Can you work these out from the model? Positions are in its coordinate system, mm. A direction names the side the tool comes from. Give positions to 0.01 mm unless a question says otherwise; leave off trailing zeros. Write each loop counter-clockwise with the first axis right and the second up, starting at its lowest first coordinate (ties: lowest second). Pieces come first, ordered by that corner, then holes. Notation, with made-up numbers: M 86.25,-31 L 131.25,-31 A19 cw 131.25,-12 Z; hole C 18,37.5 d3. An arc over 180 degrees is marked long. Use CSV: the item, a comma, the result in double quotes. Start each with the question number.
from build123d import *

# Parameters (mm, degrees)
EXTRUDE_2_DEPTH          = 35
EXTRUDE_START            = -100
SKETCH_3_W               = 70
SKETCH_3_H               = 70
EXTRUDE_3_DEPTH          = 10
CUT_EXTRUDE_START        = 35
SKETCH_4_W               = 29.4
SKETCH_4_H               = 90
CUT_EXTRUDE_1_DEPTH      = 25
CHAMFER_1_SIZE           = 10
EXTRUDE_4_DEPTH          = 15
CHAMFER_2_SIZE           = 5
CUT_EXTRUDE_2_DEPTH      = 131.096118313
CUT_EXTRUDE_2_DEPTH_BACK = 131.096118313
SKETCH_6_R               = 2
FILLET_2_R               = 8


with BuildPart() as part:
    # 草图2 → 凸台-拉伸2 (new body)
    with BuildSketch(Plane.XY):
        Polygon((-45, 7.5), (45, 7.5), (45, -12), (40, -12), (40, 0), (14.7, 0), (14.7, -100), (-14.7, -100), (-14.7, 0), (-40, 0), (-40, -12), (-45, -12), align=None)
    extrude(amount=EXTRUDE_2_DEPTH)

    # 草图3 → 凸台-拉伸3 (add)
    with BuildSketch(Plane(origin=(0, 0, 0), x_dir=(1, 0, 0), z_dir=(0, 1, 0)).offset(EXTRUDE_START)):
        with Locations((0, -35)):
            Rectangle(SKETCH_3_W, SKETCH_3_H)
    extrude(amount=EXTRUDE_3_DEPTH)

    # 草图4 → 切除-拉伸1 (cut)
    with BuildSketch(Plane.XY.offset(CUT_EXTRUDE_START)):
        with Locations((0, -45)):
            Rectangle(SKETCH_4_W, SKETCH_4_H)
    extrude(amount=-CUT_EXTRUDE_1_DEPTH, mode=Mode.SUBTRACT)

    # 倒角1
    chamfer_1_edges = [part.edges().sort_by_distance(p)[0] for p in [
        (0, 0, 10),
        (0, -90, 10),
    ]]
    chamfer(chamfer_1_edges, length=CHAMFER_1_SIZE)

    # 草图5 → 凸台-拉伸4 (add)
    with BuildSketch(Plane.XY):
        Polygon((40, -12), (45, -12), (45, 7.5), (-45, 7.5), (-45, -12), (-40, -12), (-40, 0), (40, 0), align=None)
    extrude(amount=-EXTRUDE_4_DEPTH)

    # 倒角2
    chamfer_2_edges = [part.edges().sort_by_distance(p)[0] for p in [
        (0, 0, 0),
    ]]
    chamfer(chamfer_2_edges, length=CHAMFER_2_SIZE)

    # 草图6 → 切除-拉伸2 (cut, two sides: drawn at the far end of the back side and taken through both)
    with BuildSketch(Plane(origin=(0, 0, 0), x_dir=(0, 0, -1), z_dir=(1, 0, 0)).offset(-CUT_EXTRUDE_2_DEPTH_BACK)):
        with Locations((10, -6)):
            Circle(SKETCH_6_R)
        with Locations((-25, -6)):
            Circle(SKETCH_6_R)
    extrude(amount=CUT_EXTRUDE_2_DEPTH + CUT_EXTRUDE_2_DEPTH_BACK, mode=Mode.SUBTRACT)

    # 圆角2
    fillet_2_edges = [part.edges().sort_by_distance(p)[0] for p in [
        (35, -95, 0),
        (-35, -95, 0),
        (-35, -95, 70),
        (35, -95, 70),
    ]]
    fillet(fillet_2_edges, radius=FILLET_2_R)


solid = part.part
(1) Will these pins go through, and if not, where does the flat tip stop? pin 1 Ø10 at (y, z) = (-83, 56) entering from -X; pin 2 Ø20 at (y, z) = (-38.5, 7.5) entering from +X; pin 3 Ø5 at (y, z) = (-97, 39) entering from +X; pin 4 Ø1.5 at (x, z) = (42, 18.5) entering from -Y.
(2) Which directions (+Z, -Z, +X, -X, +Y, -Y) give clear straight access to the entire face, cutting with the end or side of a thin tool? Please do faces 4 (the face through (35, -95, 35)), 5 (the face through (-35, -95, 35)), 6 (the face through (-32.594, -94.93, 2.281)), 7 (the face through (0, -3, -2)), 8 (the face through (1, 2, 35)).
(3) I want a section at C-C (z = -10). Write out the boundary of the cut face in (x, y).
(4) I want a section at A-A (z = 25). Write out the boundary of the cut face in (x, y), and give its area (4 significant figures).
(5) I want a section at B-B (x = 19). Write out the boundary of the cut face in (y, z), and give its area (4 significant figures).
(6) Please list where these lines run through material, in increasing order: L1, parallel to Z at x = -41.15, y = -6; L2, parallel to Y at x = -41.8, z = -10; L3, parallel to Y at x = 20.5, z = 10. Write a range as [from, to].
(7) I want a section at D-D (x = -11). Write out the boundary of the cut face in (y, z), and give its area (3 significant figures).
(8) Thinking about a two-plate mould opening in Y: for faces 1 (the face through (32.594, -94.93, 2.281)), 2 (the face through (42, -12, 10)), 3 (the face through (42.5, -7.2, -8.4)), which applies, released by +Y, released by -Y, zero draft, split by the parting line, or undercut?
Geometry results:
1,pin 1,"passes through"
1,pin 2,"stops at x = 14.7"
1,pin 3,"stops at x = 35"
1,pin 4,"stops at y = -12"
2,face 4,"+Z, -Z, +X, -Y"
2,face 5,"+Z, -Z, -X, -Y"
2,face 6,"-Z, -X, -Y"
2,face 7,"-Z, -Y"
2,face 8,"+Z, +X, -X, +Y"
3,outline,"M -45,-12 L -40,-12 L -40,-8 L -45,-8 Z; M -45,-4 L -40,-4 L -40,0 L 40,0 L 40,-4 L 45,-4 L 45,7.5 L -45,7.5 Z; M 40,-12 L 45,-12 L 45,-8 L 40,-8 Z"
4,outline,"M -45,-12 L -40,-12 L -40,-8 L -45,-8 Z; M -45,-4 L -40,-4 L -40,0 L 40,0 L 40,-4 L 45,-4 L 45,7.5 L -45,7.5 Z; M -35,-100 L 35,-100 L 35,-90 L -35,-90 Z; M 40,-12 L 45,-12 L 45,-8 L 40,-8 Z"
4,area,"1,455 mm2"
5,outline,"M -100,0 L -90,0 L -90,70 L -100,70 Z; M 0,-15 L 7.5,-15 L 7.5,35 L 0,35 Z"
5,area,"1,075 mm2"
6,L1,"z = [-15, -12], [-8, 23], [27, 35]"
6,L2,"y = [-12, -8], [-4, 7.5]"
6,L3,"y = [-100, -90], [0, 7.5]"
7,outline,"M -100,0 L -5,0 L 0,-5 L 0,-15 L 7.5,-15 L 7.5,35 L 0,35 L 0,20 L -10,10 L -80,10 L -90,20 L -90,70 L -100,70 Z"
7,area,"2,090 mm2"
8,face 1,"zero draft"
8,face 2,"released by -Y"
8,face 3,"undercut"
